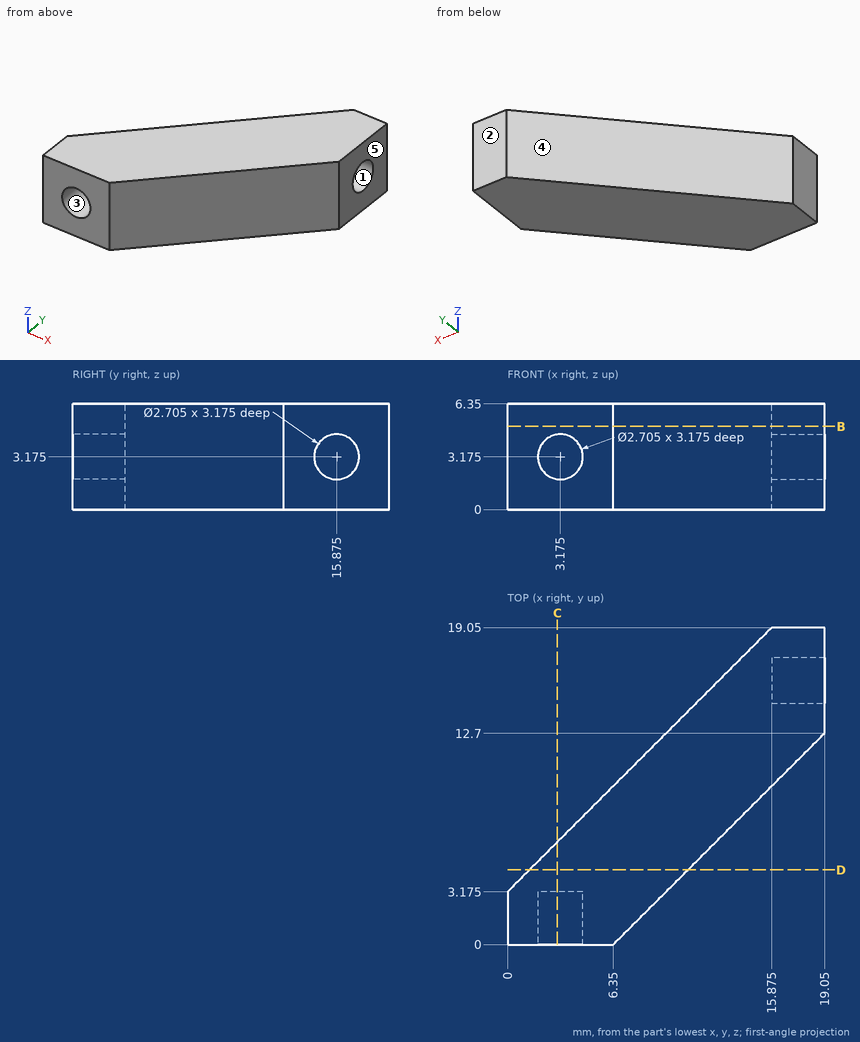
Here's the drawing with two shaded views (mm, measured from the low corner). I have some questions. A direction names the side the tool comes from. Coordinates: 2 decimals unless noted, no trailing zeros. Order: outer loops, then holes, each group sorted by start corner. A loop starts at its lowest first (then second) coordinate and runs counter-clockwise, first axis right, second up. Notation, with made-up numbers: (33.25, -8) -> (84.25, -8) arc R29 ccw to (84.25, 20) -> close; hole circle Ø10 at (22, -23). An arc over 180 degrees is marked (long way). Write each question's results on one line, items separated by ' | '.
Item 1: If we mould it in two halves opening along X, with no side actions, what happens to the marked faces 3, 4 and 5? For each: +X half, -X half, draft (parallel to the pull), parting line (faces both ways), or undercut.
Results are:
face 3: undercut | face 4: -X half | face 5: +X half
Item 2: I want a section at D-D, the plane y = 4.5. Write out the boundary of the cut face in (x, z) (3 decimals).
Results are:
outline: (1.325, 0) -> (10.85, 0) -> (10.85, 6.35) -> (1.325, 6.35) -> close
Item 3: I want a section at C-C, the plane x = 3. Write out the boundary of the cut face in (y, z) (3 decimals), then the cut area to 3 significant figures.
Results are:
outline: (0, 0) -> (6.175, 0) -> (6.175, 6.35) -> (0, 6.35) -> (0, 4.516) -> (3.175, 4.516) -> (3.175, 1.834) -> (0, 1.834) -> close | area: 30.7 mm²
Item 4: Which directions (+Z, -Z, +X, -X, +Y, -Y) give clear straight access to the entire face, cutting with the end or side of a thin tool? Please do the marked faces 1 and 2.
Results are:
face 1: +X | face 2: +Z, -Z, +X, -X, +Y
Item 5: If I drill on line 1 along Z through (x, y) = (16.5, 15); line 2 along X through (y, z) = (2.25, 2.75); line 3 along Y through (x, z) = (17, 0.5), over which ranges is the centre line in solid material (lowest first)?
Results are:
line 1: 0 to 2.14, 4.21 to 6.35 | line 2: 0 to 1.89, 4.46 to 8.6 | line 3: 10.65 to 19.05
Item 6: I'm going to push flat-ended pins straight in: pin 1 Ø1.5 at (y, z) = (9, 5.5) entering from +X; pin 2 Ø2 at (y, z) = (15.875, 3.175) entering from +X (3 decimals); pin 3 Ø3 at (x, z) = (3.5, 2.5) entering from -Y. Where does each tip first touch, or does it pass through?
Results are:
pin 1: x = 16.1 | pin 2: x = 15.875 | pin 3: y = 0
Item 7: I want a section at B-B, the plane z = 5. Write out the boundary of the cut face in (x, y) (3 decimals), then the cut area to 3 significant figures.
Results are:
outline: (0, 0) -> (6.35, 0) -> (19.05, 12.7) -> (19.05, 19.05) -> (15.875, 19.05) -> (0, 3.175) -> close | area: 156 mm²
